Input: part model. Units: mm. Frame: model coordinates. Face numbers are marked on the shaded views. Round coordinates to 2 decimals unless told otherwise and drop trailing zeros. Loops run counter-clockwise (first coordinate to the right, second up) from the corner with the lowest first, then second, coordinate; pieces in that order, holes last. Notation, with made-up numbers: (3, -20.5) -> (32, -20.5) arc R18 cw to (32, -15.5) -> close; hole circle Ø1 at (-1, 25.5). An arc over 180 degrees is marked (long way). Answer in a Markdown table with one row per item. Add a question column.
Q1. Section B-B, the plane x = -19. Output: boundary loops of the cut face in (y, z), and give its area (3 significant figures).
Q2. Ray query, L1, parallel to X at y = 22.4, z = 25; L2, parallel to X at y = 10.5, z = 125; L3, parallel to Y at x = -21, z = 49. Return the intervals inside material, ascending. Write a range as from..to.
Q3. Mould query, pull axis Y, two halves, no side actions, for the marked faces 1, 2 and 3. Classes: pulls with the +Y half, pulls with the -Y half, needs draft (parallel to the pull), parting line crosses it, or undercut.
Q4. Pin query (flat end, axial travel): pin 1 (22 mm diameter, centred on x = 1, z = 27.5, fed in from +Y); pin 2 (4 mm diameter, centred on x = -8, y = -15.5, fed in from -Z); pin 3 (16 mm diameter, centred on x = 0, z = 25, fed in from -Y); pin 4 (2 mm diameter, centred on x = -12.5, z = 85.5, fed in from +Y). Return the tip coordinate at first contact, or that it passes through.
Q5. Section A-A, the plane y = -10.5. Output: boundary loops of the cut face in (x, z).
```python
from build123d import *

# Parameters (mm, degrees)
SKIZZE1_W                       = 50
SKIZZE1_H                       = 50
AUFSATZ_LINEAR_AUSTRAGEN1_DEPTH = 150
SKIZZE2_W                       = 50
SKIZZE2_H                       = 50
AUFSATZ_LINEAR_AUSTRAGEN2_DEPTH = 1
SCHNITT_LINEAR_AUSTRAGEN1_DEPTH = 1
SCHNITT_LINEAR_AUSTRAGEN2_DEPTH = 50
SKIZZE5_R                       = 5
SCHNITT_LINEAR_AUSTRAGEN3_DEPTH = 75
SKIZZE6_R                       = 10
SCHNITT_LINEAR_AUSTRAGEN4_DEPTH = 6
SCHNITT_LINEAR_START            = -6
SKIZZE7_R                       = 10
SCHNITT_LINEAR_AUSTRAGEN5_DEPTH = 6
SKIZZE8_R                       = 21.1
SKIZZE8_R_2                     = 12.4
SCHNITT_LINEAR_AUSTRAGEN6_DEPTH = 5


with BuildPart() as part:
    # Skizze1 → Aufsatz-Linear austragen1 (new body)
    with BuildSketch(Plane.XY):
        Rectangle(SKIZZE1_W, SKIZZE1_H)
    extrude(amount=AUFSATZ_LINEAR_AUSTRAGEN1_DEPTH)

    # Skizze2 → Aufsatz-Linear austragen2 (add)
    with BuildSketch(Plane(origin=(0, 25, 0), x_dir=(1, 0, 0), z_dir=(0, 1, 0))):
        with Locations((0, -125)):
            Rectangle(SKIZZE2_W, SKIZZE2_H)
        with Locations((0, -25)):
            Rectangle(SKIZZE2_W, SKIZZE2_H)
    extrude(amount=AUFSATZ_LINEAR_AUSTRAGEN2_DEPTH)

    # Skizze3 → Schnitt-Linear austragen1 (cut)
    with BuildSketch(Plane(origin=(0, 26, 0), x_dir=(1, 0, 0), z_dir=(0, 1, 0))):
        with BuildLine():
            Line((4.2e-08, 0), (-25, 0))
            Line((-25, 0), (-25, -25))
            ThreePointArc((-25, -25), (-17.677669515, -7.322330455), (4.2e-08, 0))
        make_face()
        with BuildLine():
            Line((25, 0), (4.2e-08, 0))
            ThreePointArc((4.2e-08, 0), (17.677669545, -7.322330485), (25, -25))
            Line((25, -25), (25, 0))
        make_face()
        with BuildLine():
            Line((25, -150), (25, -125))
            ThreePointArc((25, -125), (17.67766955, -142.677669509), (5.8e-08, -150))
            Line((5.8e-08, -150), (25, -150))
        make_face()
        with BuildLine():
            ThreePointArc((5.8e-08, -150), (-17.677669509, -142.67766955), (-25, -125))
            Line((-25, -125), (-25, -150))
            Line((-25, -150), (5.8e-08, -150))
        make_face()
        with BuildLine():
            Line((-3.2e-08, -100), (-25, -100))
            Line((-25, -100), (-25, -125))
            ThreePointArc((-25, -125), (-17.677669541, -107.322330482), (-3.2e-08, -100))
        make_face()
        with BuildLine():
            Line((25, -100), (-3.2e-08, -100))
            ThreePointArc((-3.2e-08, -100), (17.677669518, -107.322330459), (25, -125))
            Line((25, -125), (25, -100))
        make_face()
        with BuildLine():
            ThreePointArc((0, -50), (-17.67766953, -42.67766953), (-25, -25))
            Line((-25, -25), (-25, -50))
            Line((-25, -50), (0, -50))
        make_face()
        with BuildLine():
            Line((25, -50), (25, -25))
            ThreePointArc((25, -25), (17.67766953, -42.67766953), (0, -50))
            Line((0, -50), (25, -50))
        make_face()
    extrude(amount=-SCHNITT_LINEAR_AUSTRAGEN1_DEPTH, mode=Mode.SUBTRACT)

    # Skizze4 → Schnitt-Linear austragen2 (cut)
    with BuildSketch(Plane(origin=(0, 25, 0), x_dir=(1, 0, 0), z_dir=(0, 1, 0))):
        with BuildLine():
            Line((25, -150), (25, -125))
            ThreePointArc((25, -125), (17.677669466, -142.677669593), (-1.79e-07, -150))
            Line((-1.79e-07, -150), (25, -150))
        make_face()
        with BuildLine():
            Line((-25, 0), (-25, -25))
            ThreePointArc((-25, -25), (-17.67766955, -7.322330491), (-5.8e-08, 0))
            Line((-5.8e-08, 0), (-25, 0))
        make_face()
        with BuildLine():
            ThreePointArc((-5.8e-08, 0), (17.677669509, -7.32233045), (25, -25))
            Line((25, -25), (25, 0))
            Line((25, 0), (-5.8e-08, 0))
        make_face()
        with BuildLine():
            ThreePointArc((-1.79e-07, -150), (-17.677669593, -142.677669466), (-25, -125))
            Line((-25, -125), (-25, -150))
            Line((-25, -150), (-1.79e-07, -150))
        make_face()
    extrude(amount=-SCHNITT_LINEAR_AUSTRAGEN2_DEPTH, mode=Mode.SUBTRACT)

    # Skizze5 → Schnitt-Linear austragen3 (cut)
    with BuildSketch(Plane(origin=(0, 26, 0), x_dir=(1, 0, 0), z_dir=(0, 1, 0))):
        with Locations(Location((0, -25, 0), (0, 0, 270))):
            Circle(SKIZZE5_R)
        with Locations(Location((0, -125, 0), (0, 0, 270))):
            Circle(SKIZZE5_R)
    extrude(amount=-SCHNITT_LINEAR_AUSTRAGEN3_DEPTH, mode=Mode.SUBTRACT)

    # Skizze6 → Schnitt-Linear austragen4 (cut)
    with BuildSketch(Plane(origin=(0, 26, 0), x_dir=(1, 0, 0), z_dir=(0, 1, 0))):
        with Locations(Location((0, -125, 0), (0, 0, 270))):
            Circle(SKIZZE6_R)
        with Locations(Location((0, -25, 0), (0, 0, 270))):
            Circle(SKIZZE6_R)
    extrude(amount=-SCHNITT_LINEAR_AUSTRAGEN4_DEPTH, mode=Mode.SUBTRACT)

    # Skizze7 → Schnitt-Linear austragen5 (cut)
    with BuildSketch(Plane.XZ.offset(25).offset(SCHNITT_LINEAR_START)):
        with Locations(Location((0, 125, 0), (0, 0, 90))):
            Circle(SKIZZE7_R)
        with Locations(Location((0, 25, 0), (0, 0, 90))):
            Circle(SKIZZE7_R)
    extrude(amount=SCHNITT_LINEAR_AUSTRAGEN5_DEPTH, mode=Mode.SUBTRACT)

    # Skizze8 → Schnitt-Linear austragen6 (cut)
    # profile 1 of 2: a face of its own
    with BuildSketch(Plane(origin=(0, 26, 0), x_dir=(1, 0, 0), z_dir=(0, 1, 0))):
        with Locations(Location((0, -25, 0), (0, 0, 270))):
            Circle(SKIZZE8_R)
        with Locations(Location((0, -25, 0), (0, 0, 270))):
            Circle(SKIZZE8_R_2, mode=Mode.SUBTRACT)
    # profile 2 of 2: a face of its own
    with BuildSketch(Plane(origin=(0, 26, 0), x_dir=(1, 0, 0), z_dir=(0, 1, 0))):
        with Locations(Location((0, -125, 0), (0, 0, 90))):
            Circle(SKIZZE8_R)
        with Locations(Location((0, -125, 0), (0, 0, 90))):
            Circle(SKIZZE8_R_2, mode=Mode.SUBTRACT)
    extrude(amount=-SCHNITT_LINEAR_AUSTRAGEN6_DEPTH, mode=Mode.SUBTRACT)


solid = part.part
```
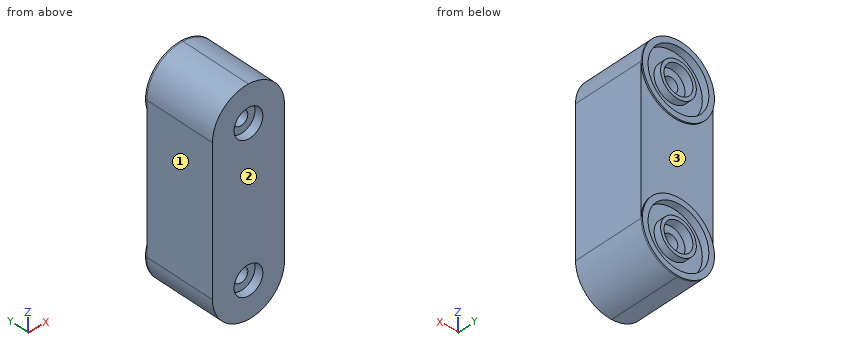
Answer block:
| question | item | result |
|---|---|---|
| 1 | outline | (-25, 8.75) -> (26, 8.75) -> (26, 15.82) -> (21, 15.82) -> (21, 34.18) -> (26, 34.18) -> (26, 41.25) -> (25, 41.25) -> (25, 108.75) -> (26, 108.75) -> (26, 115.82) -> (21, 115.82) -> (21, 134.18) -> (26, 134.18) -> (26, 141.25) -> (-25, 141.25) -> close |
| 1 | area | 6,510 mm^2 |
| 2 | L1 | -25..-21.1, -12.4..-10, 10..12.4, 21.1..25 |
| 2 | L2 | -25..-5, 5..25 |
| 2 | L3 | -25..25 |
| 3 | face 1 | needs draft |
| 3 | face 2 | pulls with the -Y half |
| 3 | face 3 | pulls with the +Y half |
| 4 | pin 1 | y = 26 |
| 4 | pin 2 | z = 0.73 |
| 4 | pin 3 | y = -19 |
| 4 | pin 4 | y = 25 |
| 5 | outline | (-25, 25) arc R25 ccw to (25, 25) -> (25, 125) arc R25 ccw to (-25, 125) -> close; hole circle Ø10 at (0, 25); hole circle Ø10 at (0, 125) |
